For this review, take the finished solid that the model builds, in its own axes (mm). A direction names the side the tool comes from. Round coordinates to 2 decimals unless told otherwise and drop trailing zeros. Order: outer loops, then holes, each group sorted by start corner. A loop starts at its lowest first (then second) coordinate and runs counter-clockwise, first axis right, second up. Notation, with made-up numbers: M 43.25,53.25 L 74.25,53.25 A22 cw 74.25,81.25 Z; hole C -4,56 d4. An arc over 180 degrees is marked long. Answer as a JSON object with one key per item and string values.
from build123d import *

# Parameters (mm, degrees)
BOSS_EXTRUDE1_DEPTH   = 10
SKETCH2_R             = 3
CUT_EXTRUDE1_DEPTH    = 10
CRVPATTERN1_OUTLINE_R = 3
CRVPATTERN1_DEPTH     = 10


# Read off the part's stored shape, not the designer's step: CrvPattern1
with BuildPart() as part:
    # Sketch1 → Boss-Extrude1 (new body)
    with BuildSketch(Plane.XY):
        with BuildLine():
            ThreePointArc((-12.160643086, -4.500395473), (-12.066298067, 4.747552068), (-5.833593115, 11.580327761))
            ThreePointArc((-5.833593115, 11.580327761), (22.801277697, 17.386949302), (50.413138808, 7.834054132))
            ThreePointArc((50.413138808, 7.834054132), (53.544482095, -9.628731125), (36.032050188, -12.46931353))
            ThreePointArc((36.032050188, -12.46931353), (25.188301018, -9.23349986), (14.747114027, -13.59687016))
            ThreePointArc((14.747114027, -13.59687016), (10.621121624, -16.149691652), (5.851758877, -17.040696634))
            ThreePointArc((5.851758877, -17.040696634), (-5.122139447, -13.59687016), (-12.160643086, -4.500395473))
        make_face()
    extrude(amount=BOSS_EXTRUDE1_DEPTH)

    # Sketch2 → Cut-Extrude1 (cut)
    with BuildSketch(Plane.XY.offset(10)):
        with Locations((5.495652988, 9.028732309)):
            Circle(SKETCH2_R)
    extrude(amount=-CUT_EXTRUDE1_DEPTH, mode=Mode.SUBTRACT)

    # CrvPattern1 outline → CrvPattern1 (cut)
    with BuildSketch(Plane.XY):
        with Locations((-5.463573367, 3.372342928)):
            Circle(CRVPATTERN1_OUTLINE_R)
        with Locations((-4.253847863, -5.460432999)):
            Circle(CRVPATTERN1_OUTLINE_R)
        with Locations((5.602614411, -10.492104281)):
            Circle(CRVPATTERN1_OUTLINE_R)
        with Locations((18.978303952, -3.768285721)):
            Circle(CRVPATTERN1_OUTLINE_R)
        with Locations((40.513825045, -7.583139488)):
            Circle(CRVPATTERN1_OUTLINE_R)
        with Locations((47.960307029, -6.163614465)):
            Circle(CRVPATTERN1_OUTLINE_R)
        with Locations((47.853730427, 1.416213148)):
            Circle(CRVPATTERN1_OUTLINE_R)
        with Locations((35.630316045, 8.091012477)):
            Circle(CRVPATTERN1_OUTLINE_R)
        with Locations((20.637040529, 10.939744191)):
            Circle(CRVPATTERN1_OUTLINE_R)
    extrude(amount=CRVPATTERN1_DEPTH, mode=Mode.SUBTRACT)


solid = part.part
1) Add section A-A on x = 42.5. State the section outline as (y, z) points, and give its area (3 significant figures).
Geometry check:
{"outline": "M -14.85,0 L -9.83,0 L -9.83,10 L -14.85,10 Z; M -5.33,0 L 12.34,0 L 12.34,10 L -5.33,10 Z", "area": "227 mm²"}
2) Add section D-D on x = 29.5. State the section outline as (y, z) points.
Geometry check:
{"outline": "M -9.56,0 L 16.53,0 L 16.53,10 L -9.56,10 Z"}
3) For L1, parallel to X at y = 4, z = 7.5; L2, parallel to X at y = -8, z = 6.5; L3, parallel to Y at x = 21.5, z = 4, list the stretches that pass through material, from the lowest coordinate up.
Geometry check:
{"L1": "x = -12.33 to -8.4, -2.53 to 46.33, 49.38 to 54.04", "L2": "x = -10.44 to -5.85, -2.66 to 3.93, 7.27 to 37.54, 43.48 to 45.59, 50.33 to 54.52", "L3": "y = -9.84 to -5.39, -2.14 to 8.07, 13.81 to 17.46"}
4) Mouldability with a two-part tool opening along Y and no side actions: class faces 3 (the cylindrical face through (-7.25, -5.33, 4.93)), 4 (the cylindrical face through (25.35, -9.226, 4.93)), 5 (the cylindrical face through (-12.114, 4.624, 4.93)) as +Y half, -Y half, draft (parallel to the pull), parting line (faces both ways), or undercut.
Geometry check:
{"face 3": "undercut", "face 4": "-Y half", "face 5": "parting line"}
5) Add section B-B on z = 3.75. State how many separate pieces and enclosed holes the cut face has, and give its area (3 significant figures).
Geometry check:
{"separate pieces": "1", "enclosed holes": "10", "area": "1,510 mm²"}
6) Add section C-C on y = 15. State the section outline as (x, z) points.
Geometry check:
{"outline": "M 2.62,0 L 35.61,0 L 35.61,10 L 2.62,10 Z"}
7) Machinability: for faces 1 (the cylindrical face through (10.685, -16.125, 4.93)), 2 (the cylindrical face through (38.4, 6.94, 4.93)), which of the approach directions +Z, -Z, +X, -X, +Y, -Y give a long, thin tool a straight path to every point of the face, cutting with its end or side? Answer none if there is none.
Geometry check:
{"face 1": "+Z, -Z, -Y", "face 2": "+Z, -Z"}
8) Insertion check: P1, Ø2, axis at y = -4, z = 2, coming from the +X side; P2, Ø4, axis at x = -2, z = 4.5, coming from the -Y side; P3, Ø2, axis at y = 4.5, z = 5.5, coming from the +X side; P4, Ø3.5, axis at x = 5.6, y = -10.49, coming from the -Z side. Each pin has a flat end and moves straight along its axis. Give the tip position at first contact, or say it passes through.
Geometry check:
{"P1": "stops at x = 55.82", "P2": "stops at y = -16.13", "P3": "stops at x = 54.33", "P4": "passes through"}
